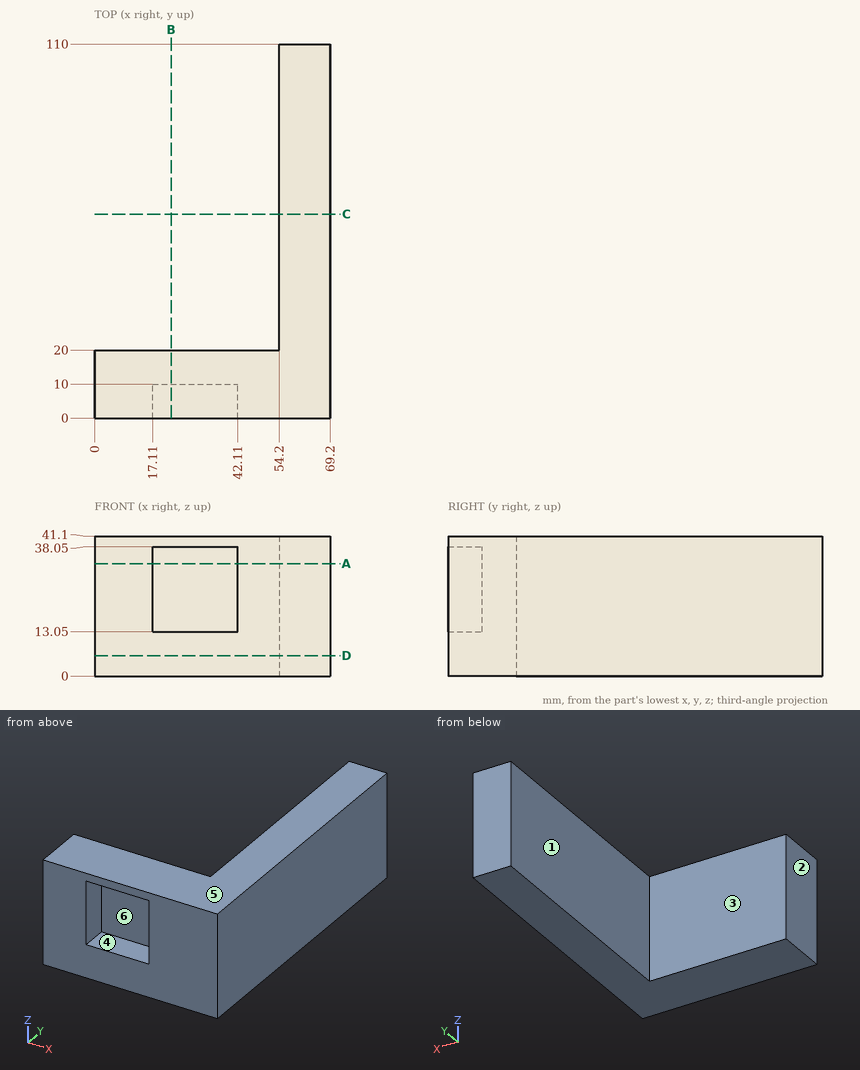
Can you work these out from the drawing? Everything is in mm from the part's minimum corner. A direction names the side the tool comes from. Coordinates: 2 decimals unless noted, no trailing zeros. Loops run counter-clockwise (first coordinate to the right, second up) from the corner with the lowest first, then second, coordinate; pieces in that order, holes last.
1) I need wall thicknesses on probe 1 along X at (y, z) = (76.5, 31); probe 2 along Y at (x, z) = (27, 32); probe 3 along Y at (x, z) = (53.5, 38.5). Which ranges of each line are inside material? Lowest first, please.
2) Thinking about a two-plate mould opening in Z: for the marked faces 3, 4, 5 and 6, which applies, pulls with the +Z half, pulls with the -Z half, needs draft (parallel to the pull), parting line crosses it, or undercut?
3) Which directions (+Z, -Z, +X, -X, +Y, -Y) give clear straight access to the entire face, cutting with the end or side of a thin tool? Please do the marked faces 1 and 2.
4) Imagine slicing it at D-D on z = 6. List the corners of the cut face in (x, y) for me.
5) Imagine slicing it at B-B on x = 22.5. List the corners of the cut face in (y, z) for me, plus the area to 3 significant figures.
6) Imagine slicing it at A-A on z = 33. List the corners of the cut face in (x, y) for me, plus the area to 3 significant figures.
7) For pin 1 (5 mm diameter, centred on x = 10, z = 32, fed in from +Y); pin 2 (2 mm diameter, centred on x = 30.5, z = 9, fed in from -Y); pin 3 (7.5 mm diameter, centred on x = 30.5, z = 30, fed in from -Y), each with a flat end and sliding along its axis, tell me the tip position at first contact or that it passes through.
8) Imagine slicing it at C-C on y = 60. List the corners of the cut face in (x, z) for me, plus the area to 4 significant figures.
Completed:
1. probe 1: x = 54.2 to 69.2
1. probe 2: y = 10 to 20
1. probe 3: y = 0 to 20
2. face 3: needs draft
2. face 4: undercut
2. face 5: pulls with the +Z half
2. face 6: undercut
3. face 1: +Z, -Z, -X, +Y
3. face 2: +Z, -Z, -X, +Y, -Y
4. outline: (0, 0) - (69.2, 0) - (69.2, 110) - (54.2, 110) - (54.2, 20) - (0, 20) - close
5. outline: (0, 0) - (20, 0) - (20, 41.1) - (0, 41.1) - (0, 38.05) - (10, 38.05) - (10, 13.05) - (0, 13.05) - close
5. area: 572 mm2
6. outline: (0, 0) - (17.11, 0) - (17.11, 10) - (42.11, 10) - (42.11, 0) - (69.2, 0) - (69.2, 110) - (54.2, 110) - (54.2, 20) - (0, 20) - close
6. area: 2,480 mm2
7. pin 1: stops at y = 20
7. pin 2: stops at y = 0
7. pin 3: stops at y = 10
8. outline: (54.2, 0) - (69.2, 0) - (69.2, 41.1) - (54.2, 41.1) - close
8. area: 616.5 mm2
